```python
from build123d import *


with BuildPart() as part:
    # 草图1 → 旋转1 (revolve)
    with BuildSketch(Plane.XY, mode=Mode.PRIVATE) as revolve_1_sk:
        with BuildLine():
            Line((-5, -9.5), (-5, 0))
            Line((-5, 0), (-6, 0))
            Line((-6, 0), (-6, 1.8))
            Line((-6, 1.8), (-4.6, 1.8))
            Line((-4.6, 1.8), (-3.9, 83.8))
            Line((-3.9, 83.8), (-2.9, 83.8))
            Line((-2.9, 83.8), (-2.9, 84.6))
            Line((-2.9, 84.6), (-3.9, 84.6))
            Line((-3.9, 84.6), (-3.9, 85.4))
            Line((-3.9, 85.4), (-2.9, 85.4))
            Line((-2.9, 85.4), (-2.9, 86.258788541))
            Line((-2.9, 86.258788541), (-3.735091076, 86.258788541))
            Line((-3.735091076, 86.258788541), (-3.735091076, 92.758788541))
            ThreePointArc((-3.735091076, 92.758788541), (-2.342754752, 94.800693716), (0, 95.587762553))
            Line((0, 95.587762553), (0, -9.5))
            Line((0, -9.5), (-5, -9.5))
        make_face()
    revolve(revolve_1_sk.sketch.rotate(Axis((0, 100.774977187, 0), (0, -1, 0)), 270), axis=Axis((0, 100.774977187, 0), (0, -1, 0)))


solid = part.part
```
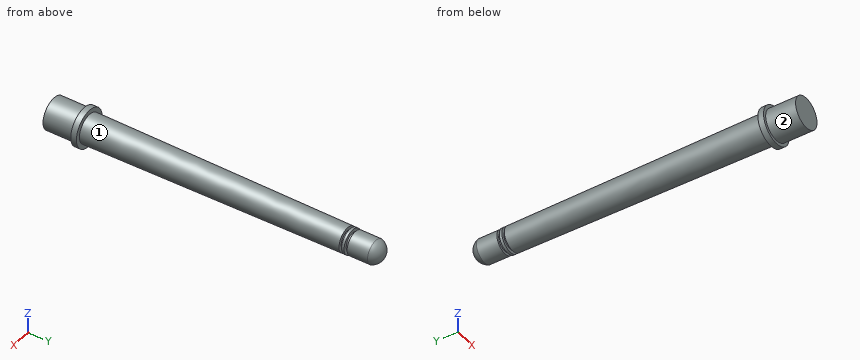
Here's how the part is built. I have some questions about the finished solid (model axes, mm). Face numbers are marked on the shaded views. A direction names the side the tool comes from. Coordinates: 2 decimals unless noted, no trailing zeros. Loops run counter-clockwise (first coordinate to the right, second up) from the corner with the lowest first, then second, coordinate; pieces in that order, holes last. Notation, with made-up numbers: (-27, -4) -> (-12, -4) arc R16 ccw to (-12, 24) -> close; hole circle Ø7 at (69, 58). An arc over 180 degrees is marked (long way). Return JSON: item names as keys, results as strings.
1) I need wall thicknesses on line 1 (Y direction, x = -2.25, z = -2.25); line 2 (Y direction, x = 3.75, z = -4.5); line 3 (Z direction, x = -1, y = 71). Which ranges of each line are inside material? Lowest first, please. Write a range as from..to.
Results below:
{"line 1": "-9.5..83.8, 84.6..85.4, 86.26..93.93", "line 2": "0..1.8", "line 3": "-3.88..3.88"}
2) Will these pins go through, and if not, where does the flat tip stop? pin 1 (1.5 mm diameter, centred on y = 10, z = 1.5, fed in from -X); pin 2 (2 mm diameter, centred on x = -4, z = -2, fed in from +Y); pin 3 (5 mm diameter, centred on x = 4, y = 75.5, fed in from +Z).
Results below:
{"pin 1": "x = -4.47", "pin 2": "y = 93.44", "pin 3": "z = 3.68"}
3) If we section it at A-A, the plane y = 74.5: Write out the boundary of the cut face in (x, z).
Results below:
{"outline": "circle Ø7.96 at (0, 0)"}
4) For the marked faces 1 and 2, which set-ups out of +Z, -Z, +X, -X, +Y, -Y let a thin tool reach every point of the face, with its end or its side?
Results below:
{"face 1": "+Y", "face 2": "-Y"}
